```python
from build123d import *

# Parameters (mm, degrees)
ESQUISSE1_W             = 34.75
ESQUISSE1_H             = 28
BOSS_EXTRU_1_DEPTH      = 8
CONG_1_R                = 4
ENL_V_MAT_EXTRU_1_DEPTH = 6
BOSS_EXTRU_2_DEPTH      = 8
CONG_2_R                = 1
CONG_1_OF_SYM_TRIE1_R   = 4
CONG_2_OF_SYM_TRIE1_R   = 1


with BuildPart() as part:
    # Esquisse1 → Boss.-Extru.1 (new body)
    with BuildSketch(Plane.XY):
        with Locations((-17.375, 0)):
            Rectangle(ESQUISSE1_W, ESQUISSE1_H)
    boss_extru_1 = extrude(amount=BOSS_EXTRU_1_DEPTH)

    # Congé1
    cong_1_edges = [part.edges().sort_by_distance(p)[0] for p in [
        (-34.75, -14, 4),
        (-34.75, 14, 4),
    ]]
    fillet(cong_1_edges, radius=CONG_1_R)

    # Esquisse3 → Enlèv. mat.-Extru.1 (cut)
    with BuildSketch(Plane.XY.offset(8)):
        with BuildLine():
            Line((0, -12.5), (0, 12.5))
            Line((0, 12.5), (-31, 12.5))
            ThreePointArc((-31, 12.5), (-33.121320344, 11.621320344), (-34, 9.5))
            Line((-34, 9.5), (-34, -9.5))
            ThreePointArc((-34, -9.5), (-33.121320344, -11.621320344), (-31, -12.5))
            Line((-31, -12.5), (0, -12.5))
        make_face()
    enl_v_mat_extru_1 = extrude(amount=-ENL_V_MAT_EXTRU_1_DEPTH, mode=Mode.SUBTRACT)

    # Esquisse5 → Boss.-Extru.2 (add)
    with BuildSketch(Plane.XY):
        Polygon((-34.75, 2.45), (-36.9, 2.45), (-36.9, 4.85), (-38.4, 4.85), (-40, 3.25), (-40, -3.25), (-38.4, -4.85), (-36.9, -4.85), (-36.9, -2.45), (-34.75, -2.45), align=None)
    boss_extru_2 = extrude(amount=BOSS_EXTRU_2_DEPTH)

    # Congé2
    cong_2_edges = [part.edges().sort_by_distance(p)[0] for p in [
        (-38.4, -4.85, 4),
        (-40, -3.25, 4),
        (-40, 3.25, 4),
        (-38.4, 4.85, 4),
        (-34.75, 2.45, 4),
        (-34.75, -2.45, 4),
    ]]
    fillet(cong_2_edges, radius=CONG_2_R)

    # Symétrie1: Boss.-Extru.1, Enlèv. mat.-Extru.1, Boss.-Extru.2 across plane
    add(boss_extru_1.mirror(Plane(origin=(0, -14, 8), x_dir=(0, 0, 1), z_dir=(-1, 0, 0))))
    add(enl_v_mat_extru_1.mirror(Plane(origin=(0, -14, 8), x_dir=(0, 0, 1), z_dir=(-1, 0, 0))), mode=Mode.SUBTRACT)
    add(boss_extru_2.mirror(Plane(origin=(0, -14, 8), x_dir=(0, 0, 1), z_dir=(-1, 0, 0))))

    # Congé1 of Symétrie1
    cong_1_of_sym_trie1_edges = [part.edges().sort_by_distance(p)[0] for p in [
        (34.75, -14, 4),
        (34.75, 14, 4),
    ]]
    fillet(cong_1_of_sym_trie1_edges, radius=CONG_1_OF_SYM_TRIE1_R)

    # Congé2 of Symétrie1
    cong_2_of_sym_trie1_edges = [part.edges().sort_by_distance(p)[0] for p in [
        (38.4, -4.85, 4),
        (40, -3.25, 4),
        (40, 3.25, 4),
        (38.4, 4.85, 4),
        (34.75, 2.45, 4),
        (34.75, -2.45, 4),
    ]]
    fillet(cong_2_of_sym_trie1_edges, radius=CONG_2_OF_SYM_TRIE1_R)


solid = part.part
```
Geometry check sheet. Reference: the model listing, model coordinates, mm. A direction names the side the tool comes from. Round coordinates to 2 decimals unless told otherwise and drop trailing zeros. Loops run counter-clockwise (first coordinate to the right, second up) from the corner with the lowest first, then second, coordinate; pieces in that order, holes last. Notation, with made-up numbers: M -40,-25 L -17,-25 A20 ccw -17,-20 Z; hole C 64,78.5 d2. An arc over 180 degrees is marked long. Return JSON: item names as keys, results as strings. Group by question number.
(1) Section check A-A, the plane x = -1. Enter the section's corners in (y, z).
(2) Mould release check, pull along X, two halves, no side actions. Record for faces 6 (the face through (0, 12.5, 5)), 7 (the face through (-33.609, 12.797, 4.056)), 8 (the face through (40, 0, 4)): pulls with the +X half, pulls with the -X half, needs draft (parallel to the pull), parting line crosses it, or undercut.
(3) Section check B-B, the plane y = -6.5. Enter the section's corners in (x, z), and give its area (3 significant figures).
(4) Go/stop test with flat-tipped pins: pin 1 (0.7 mm diameter, centred on y = 4, z = 5.5, fed in from +X); pin 2 (1.3 mm diameter, centred on x = 36, z = 3, fed in from -Y); pin 3 (0.9 mm diameter, centred on x = -36.5, z = 4, fed in from -Y). Record where each tip stops, or that it passes through.
(5) Scan lines: line 1 along X through (y, z) = (-9.5, 7.75); line 2 along Y through (x, z) = (15.5, 4.75); line 3 along X through (y, z) = (-1.5, 6). Record each from-to range of solid material in increasing order. Write a range as [from, to].
(6) Set-up check for faces 1 (the face through (-33.14, -11.6, 5.04)), 2 (the face through (-36.9, -4, 4)), 3 (the face through (3, 13, 8)), 4 (the face through (0, 14, 4)), 5 (the face through (36.9, 4, 4)): record each of +Z, -Z, +X, -X, +Y, -Y from which the full face is reachable in a straight line by a thin tool's end or side.
Data:
{
 "1": {"outline": "M -14,0 L 14,0 L 14,8 L 12.5,8 L 12.5,2 L -12.5,2 L -12.5,8 L -14,8 Z"},
 "2": {"face 6": "undercut", "face 7": "pulls with the -X half", "face 8": "pulls with the +X half"},
 "3": {"outline": "M -34.75,0 L 34.75,0 L 34.75,8 L 34,8 L 34,2 L -34,2 L -34,8 L -34.75,8 Z", "area": "148 mm²"},
 "4": {"pin 1": "x = 39.6", "pin 2": "y = -2.53", "pin 3": "y = -4.85"},
 "5": {"line 1": "[-34.75, -34], [34, 34.75]", "line 2": "[-14, -12.5], [12.5, 14]", "line 3": "[-40, -34], [34, 40]"},
 "6": {"face 1": "+Z", "face 2": "+Z, -Z, -Y", "face 3": "+Z, +X, -X, +Y, -Y", "face 4": "+Z, -Z, +X, -X, +Y", "face 5": "+Z, -Z, +Y"}
}
